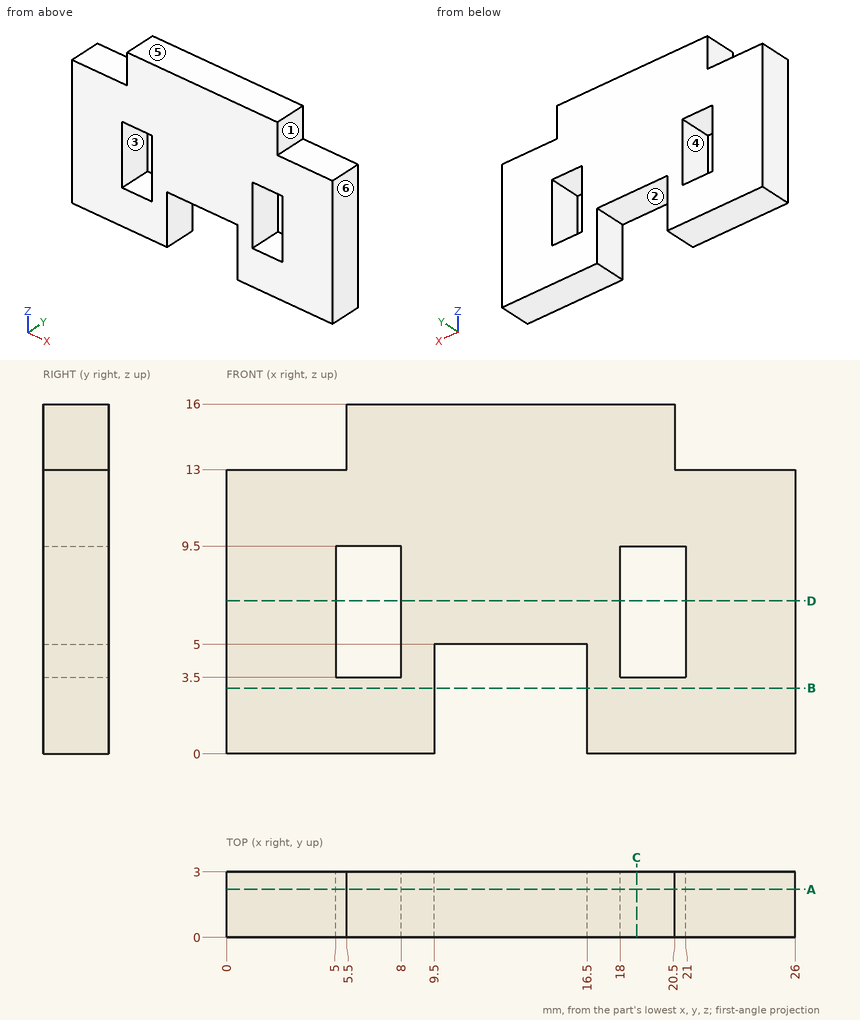
Source: three-view drawing plus pictorial views. Frame: mm from the lowest corner of the part. A direction names the side the tool comes from. Round coordinates to 2 decimals unless told otherwise and drop trailing zeros. Write each loop counter-clockwise with the first axis right and the second up, starting at its lowest first coordinate (ties: lowest second). Pieces come first, ordered by that corner, then holes. Notation, with made-up numbers: (-20, -26) -> (13, -26) arc R34 ccw to (13, 9) -> close; hole circle Ø6 at (40.5, -39.75). An arc over 180 degrees is marked (long way). Return JSON: item names as keys, results as strings.
Q1. Section A-A on y = 2.2. Return the cut outline in (x, z), and give its area (3 significant figures).
From the geometry:
{"outline": "(0, 0) -> (9.5, 0) -> (9.5, 5) -> (16.5, 5) -> (16.5, 0) -> (26, 0) -> (26, 13) -> (20.5, 13) -> (20.5, 16) -> (5.5, 16) -> (5.5, 13) -> (0, 13) -> close; hole (5, 3.5) -> (8, 3.5) -> (8, 9.5) -> (5, 9.5) -> close; hole (18, 3.5) -> (21, 3.5) -> (21, 9.5) -> (18, 9.5) -> close", "area": "312 mm2"}
Q2. Ray query, line 1 (X direction, y = 0.65, z = 6.5); line 2 (X direction, y = 2.25, z = 2.5); line 3 (Z direction, x = 19, y = 1.7). Return the intervals inside material, ascending.
From the geometry:
{"line 1": "0 to 5, 8 to 18, 21 to 26", "line 2": "0 to 9.5, 16.5 to 26", "line 3": "0 to 3.5, 9.5 to 16"}
Q3. Set-up query: the marked faces 1, 2 and 3. Return all of +Z, -Z, +X, -X, +Y, -Y with unobstructed straight access to the full face (end or side cutting, diameter ignored); none if empty.
From the geometry:
{"face 1": "+Z, +X, +Y, -Y", "face 2": "-Z, +Y, -Y", "face 3": "+Y, -Y"}
Q4. Mould query, pull axis X, two halves, no side actions, for the marked faces 4, 5 and 6. Classes: +X half, -X half, draft (parallel to the pull), parting line (faces both ways), or undercut.
From the geometry:
{"face 4": "undercut", "face 5": "draft", "face 6": "+X half"}
Q5. Section B-B on z = 3. Return the cut outline in (x, y), and give its area (3 significant figures).
From the geometry:
{"outline": "(0, 0) -> (9.5, 0) -> (9.5, 3) -> (0, 3) -> close; (16.5, 0) -> (26, 0) -> (26, 3) -> (16.5, 3) -> close", "area": "57.0 mm2"}
Q6. First-contact query: pin 1 Ø1.5 at (x, y) = (13, 1) entering from -Z; pin 2 Ø1.5 at (x, y) = (22.5, 2) entering from +Z. Flat tips, straight axial feed; report the tip coordinate or a pass-through.
From the geometry:
{"pin 1": "z = 5", "pin 2": "z = 13"}
Q7. Section D-D on z = 7. Return the cut outline in (x, y), and give its area (3 significant figures).
From the geometry:
{"outline": "(0, 0) -> (5, 0) -> (5, 3) -> (0, 3) -> close; (8, 0) -> (18, 0) -> (18, 3) -> (8, 3) -> close; (21, 0) -> (26, 0) -> (26, 3) -> (21, 3) -> close", "area": "60.0 mm2"}
Q8. Section C-C on x = 18.75. Return the cut outline in (y, z).
From the geometry:
{"outline": "(0, 0) -> (3, 0) -> (3, 3.5) -> (0, 3.5) -> close; (0, 9.5) -> (3, 9.5) -> (3, 16) -> (0, 16) -> close"}
